Design review of the part built by this model. Coordinates are the model's own, in mm. A direction names the side the tool comes from. Give positions to 0.01 mm unless a question says otherwise; leave off trailing zeros. Write each loop counter-clockwise with the first axis right and the second up, starting at its lowest first coordinate (ties: lowest second). Pieces come first, ordered by that corner, then holes. Notation, with made-up numbers: M 86.5,70 L 143.5,70 A25 cw 143.5,100 Z; hole C -1.5,-7 d11. An arc over 180 degrees is marked long. Use one line per item in the form item = value. Start each with the question number.
from build123d import *

# Parameters (mm, degrees)
BASE_EXTRUDE_DEPTH  = 3.81
SKETCH2_R           = 14.986
BOSS_EXTRUDE1_DEPTH = 15.875
SKETCH3_R           = 12.7
CUT_EXTRUDE1_DEPTH  = 20.685


with BuildPart() as part:
    # Sketch1 → Base-Extrude (new body)
    with BuildSketch(Plane(origin=(0, 0, 0), x_dir=(1, 0, 0), z_dir=(0, 1, 0))):
        with BuildLine():
            Line((-10.414, 20.574), (10.414, 20.574))
            ThreePointArc((10.414, 20.574), (17.598204897, 17.598204897), (20.574, 10.414))
            Line((20.574, 10.414), (20.574, -10.414))
            ThreePointArc((20.574, -10.414), (17.598204897, -17.598204897), (10.414, -20.574))
            Line((10.414, -20.574), (-10.414, -20.574))
            ThreePointArc((-10.414, -20.574), (-17.598204897, -17.598204897), (-20.574, -10.414))
            Line((-20.574, -10.414), (-20.574, 10.414))
            ThreePointArc((-20.574, 10.414), (-17.598204897, 17.598204897), (-10.414, 20.574))
        make_face()
    extrude(amount=BASE_EXTRUDE_DEPTH)

    # Sketch2 → Boss-Extrude1 (add)
    with BuildSketch(Plane(origin=(0, 3.81, 0), x_dir=(-1, 0, 0), z_dir=(0, 1, 0))):
        Circle(SKETCH2_R)
    extrude(amount=BOSS_EXTRUDE1_DEPTH)

    # Sketch3 → Cut-Extrude1 (cut, through all)
    with BuildSketch(Plane(origin=(0, 19.685, 0), x_dir=(-1, 0, 0), z_dir=(0, 1, 0))):
        Circle(SKETCH3_R)
    extrude(amount=-CUT_EXTRUDE1_DEPTH, mode=Mode.SUBTRACT)


solid = part.part
1. We need section A-A (z = 0). State the section outline as (x, y) points (3 decimals).
2. For faces 4 (the flat face through (9, 3.81, -14)), 5 (the flat face through (-20.574, 2, 0)), list the 3-axis set-ups (+Z, -Z, +X, -X, +Y, -Y) from which the entire face can be reached by the end or side of a thin tool; tool diameter is ignored.
3. To check wall thickness, follow L1, parallel to Z at x = 0, y = 12.5; L2, parallel to Y at x = 10.5, z = 17; L3, parallel to X at y = 7, z = 1. State the ranges of each line that lie inside material, in increasing order.
4. We need section C-C (y = 10.5). State the section outline as (x, z) points.
5. We need section B-B (x = 0). State the section outline as (y, z) points (3 decimals).
6. Draft analysis for pull direction Z (two halves, no side actions). For faces 1 (the cylindrical face through (17.677, 1.878, 17.519)), 2 (the cylindrical face through (2.75, 9.98, -12.4)), 3 (the flat face through (9.4, 0, -9.4)), state which applies: pulls with the +Z half, pulls with the -Z half, needs draft (parallel to the pull), parting line crosses it, or undercut.
7. Clearance check with flat-ended pins moving along their axes: pin 1 Ø5 at (x, y) = (-14.5, 7.5) entering from +Z; pin 2 Ø1 at (x, y) = (7.5, 13.5) entering from -Z; pin 3 Ø2 at (y, z) = (17.5, -8) entering from +X; pin 4 Ø6 at (x, z) = (12, 11) entering from -Y. State where each tip first meets the part, or that it passes through.
8. We need section D-D (z = -14). State the section outline as (x, y) points (3 decimals).
Answer block:
q1.outline = M -20.574,0 L -12.7,0 L -12.7,19.685 L -14.986,19.685 L -14.986,3.81 L -20.574,3.81 Z; M 12.7,0 L 20.574,0 L 20.574,3.81 L 14.986,3.81 L 14.986,19.685 L 12.7,19.685 Z
q2.face_4 = +Y
q2.face_5 = +Z, -Z, -X, +Y, -Y
q3.L1 = -14.99 to -12.7, 12.7 to 14.99
q3.L2 = 0 to 3.81
q3.L3 = -14.95 to -12.66, 12.66 to 14.95
q4.outline = C 0,0 d29.97; hole C 0,0 d25.4
q5.outline = M 0,-20.574 L 3.81,-20.574 L 3.81,-14.986 L 19.685,-14.986 L 19.685,-12.7 L 0,-12.7 Z; M 0,12.7 L 19.685,12.7 L 19.685,14.986 L 3.81,14.986 L 3.81,20.574 L 0,20.574 Z
q6.face_1 = pulls with the +Z half
q6.face_2 = undercut
q6.face_3 = needs draft
q7.pin_1 = 8.98
q7.pin_2 = -13.25
q7.pin_3 = 13.25
q7.pin_4 = 0
q8.outline = M -19.92,0 L 19.92,0 L 19.92,3.81 L 5.346,3.81 L 5.346,19.685 L -5.346,19.685 L -5.346,3.81 L -19.92,3.81 Z
